Design review of the part shown in the three views and the two pictorial views. Dimensions are in mm from the part's minimum x, y and z. Round coordinates to 2 decimals unless told otherwise and drop trailing zeros. Write each loop counter-clockwise with the first axis right and the second up, starting at its lowest first coordinate (ties: lowest second). Pieces come first, ordered by that corner, then holes. Notation, with made-up numbers: (57.5, 33.5) -> (100.5, 33.5) arc R26 cw to (100.5, 53.5) -> close; hole circle Ø5 at (-4, 70.5). An arc over 180 degrees is marked (long way). Answer as a JSON object with one key per item and string values. Group by question number.
1) We need section B-B, the plane z = 2.7. Count the separate pieces of the cut face and the enclosed holes in it, then the cut area to 3 significant figures.
2) We need section A-A, the plane y = 32.5. Write out the cut boundary in (x, z), then the cut area to 3 significant figures.
3) We need section D-D, the plane x = 35. Write out the cut boundary in (y, z).
4) To check wall thickness, follow probe 1 along X at (y, z) = (53, 2.75); probe 2 along Y at (x, z) = (19, 3.5) (3 decimals); probe 3 along Y at (x, z) = (3.5, 1.9). State the ranges of each line that lie inside material, in increasing order. Write a range as [from, to].
5) Insertion check: pin 1 Ø3.5 at (x, y) = (30, 42.5) entering from +Z; pin 2 Ø2 at (x, z) = (34, 3) entering from -Y. Each pin has a flat end and moves straight along its axis. Give the tip position at first contact, or say it passes through.
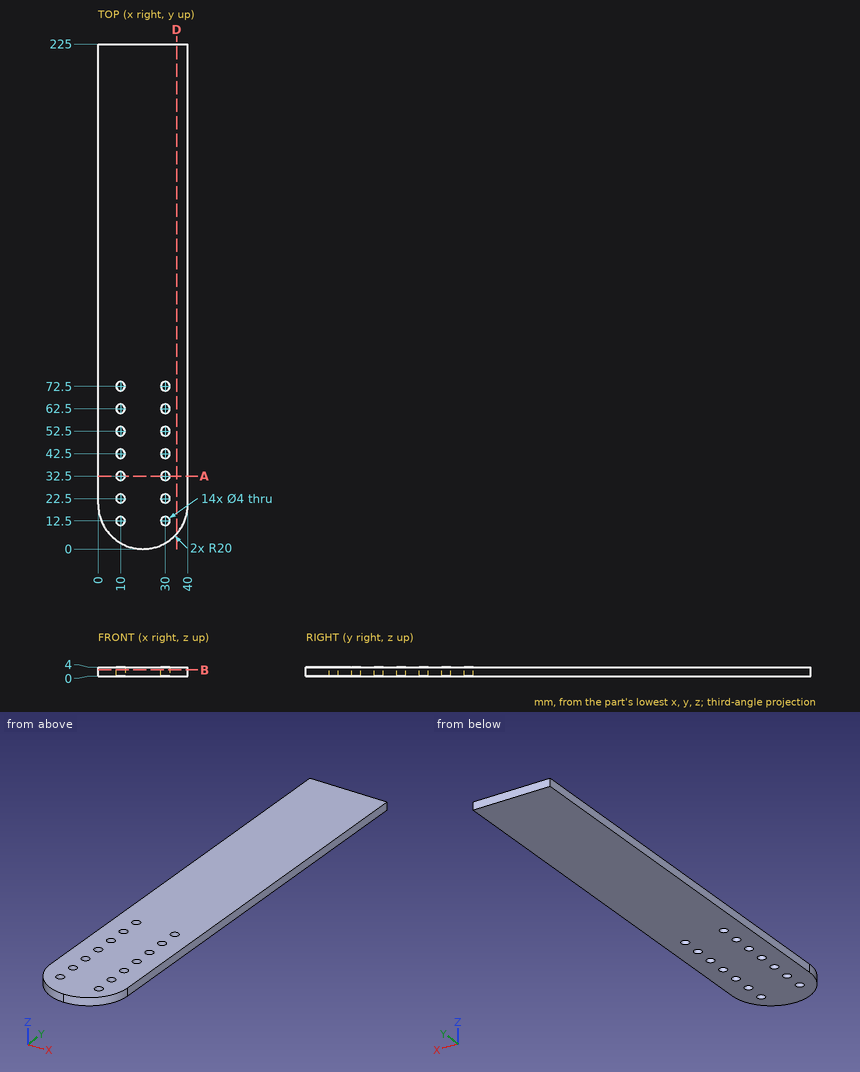
Here are the results:
{
 "1": {"separate pieces": "1", "enclosed holes": "14", "area": "8,650 mm^2"},
 "2": {"outline": "(0, 0) -> (8, 0) -> (8, 4) -> (0, 4) -> close; (12, 0) -> (28, 0) -> (28, 4) -> (12, 4) -> close; (32, 0) -> (40, 0) -> (40, 4) -> (32, 4) -> close", "area": "128 mm^2"},
 "3": {"outline": "(6.77, 0) -> (225, 0) -> (225, 4) -> (6.77, 4) -> close"},
 "4": {"probe 1": "x = [0, 8.06], [11.94, 28.06], [31.94, 40]", "probe 2": "y = [0.025, 225]", "probe 3": "y = [8.7, 225]"},
 "5": {"pin 1": "passes through", "pin 2": "stops at y = 4.8"}
}
